Here's the drawing with two shaded views (mm, measured from the low corner). I have some questions. A direction names the side the tool comes from. Give positions to 0.01 mm unless a question says otherwise; leave off trailing zeros. Write each loop counter-clockwise with the first axis right and the second up, starting at its lowest first coordinate (ties: lowest second). Pieces come first, ordered by that corner, then holes. Notation, with made-up numbers: M 52,-18.75 L 71,-18.75 A16 cw 71,-13.75 Z; hole C -19,73.5 d10. An arc over 180 degrees is marked long. Answer as a JSON object with one key per item and string values. Group by question number.
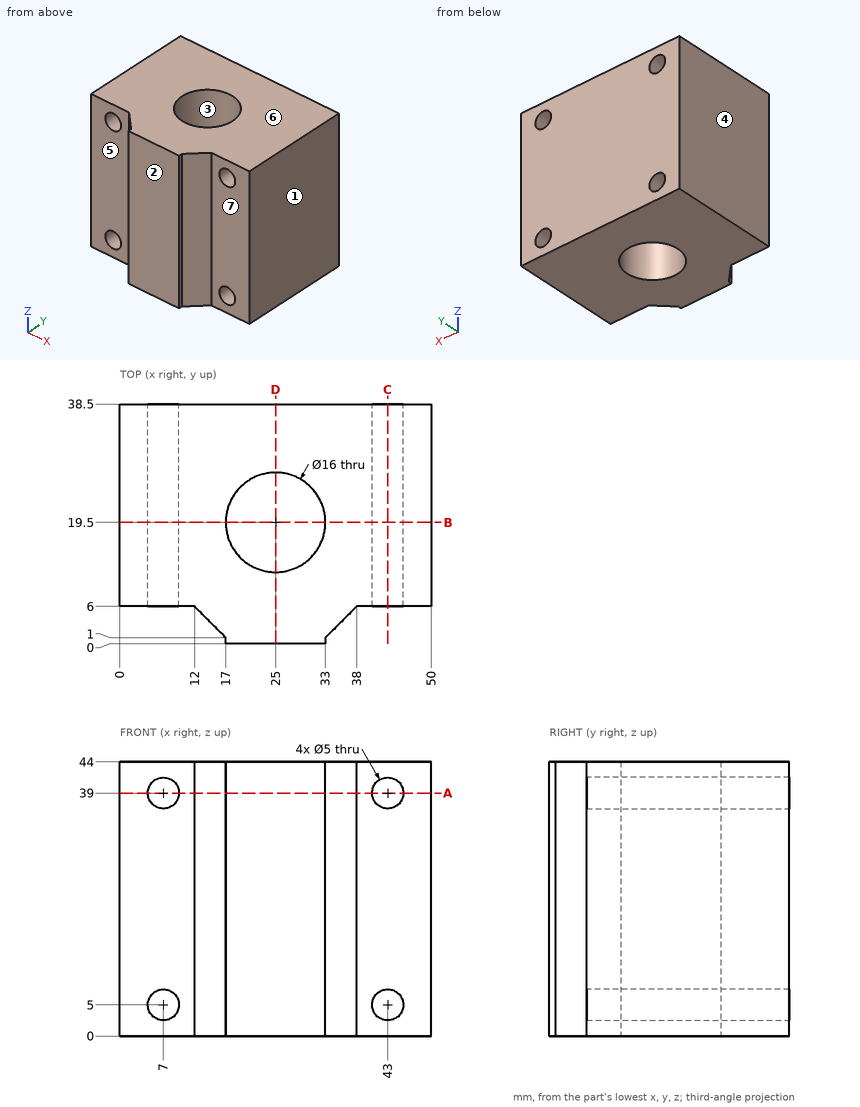
1) Please list where these lines run through material, in increasing order: line 1 along X through (y, z) = (31, 39); line 2 along X through (y, z) = (25, 39); line 3 along X through (y, z) = (18, 39.5). Write a range as from..to.
2) We'd pull the mould along X, two halves only. Please class the marked faces 1, 2, 3 and 4: released by +X, released by -X, zero draft, split by the parting line, or undercut.
3) For the marked faces 5, 6 and 7, which set-ups out of +Z, -Z, +X, -X, +Y, -Y let a thin tool reach every point of the face, with its end or its side?
4) I'm going to push flat-ended pins straight in: pin 1 (0.8 mm diameter, centred on y = 0.5, z = 24, fed in from -X); pin 2 (0.5 mm diameter, centred on y = 0.5, z = 30, fed in from +X); pin 3 (13 mm diameter, centred on x = 41.5, z = 11.5, fed in from -Y). Where does each tip first touch, or does it pass through?
5) If we section it at A-A, the plane z = 39: List the corners of the cut face in (x, y) for me, plus the area to 3 significant figures.
6) If we section it at D-D, the plane x = 25: List the corners of the cut face in (y, z) for me.
7) If we section it at B-B, the plane y = 19.5: List the corners of the cut face in (x, z) for me.
8) If we section it at C-C, the plane x = 43: List the corners of the cut face in (y, z) for me.
Taken from the geometry:
{
 "1": {"line 1": "0..4.5, 9.5..40.5, 45.5..50", "line 2": "0..4.5, 9.5..19.19, 30.81..40.5, 45.5..50", "line 3": "0..4.55, 9.45..17.14, 32.86..40.55, 45.45..50"},
 "2": {"face 1": "released by +X", "face 2": "zero draft", "face 3": "undercut", "face 4": "released by -X"},
 "3": {"face 5": "+Z, -Z, -X, -Y", "face 6": "+Z, +X, -X, +Y, -Y", "face 7": "+Z, -Z, +X, -Y"},
 "4": {"pin 1": "x = 17", "pin 2": "x = 33", "pin 3": "y = 3"},
 "5": {"outline": "M 0,6 L 4.5,6 L 4.5,38.5 L 0,38.5 Z; M 9.5,6 L 12,6 L 17,1 L 17,0 L 33,0 L 33,1 L 38,6 L 40.5,6 L 40.5,38.5 L 9.5,38.5 Z; M 45.5,6 L 50,6 L 50,38.5 L 45.5,38.5 Z; hole C 25,19.5 d16", "area": "1,220 mm²"},
 "6": {"outline": "M 0,0 L 11.5,0 L 11.5,44 L 0,44 Z; M 27.5,0 L 38.5,0 L 38.5,44 L 27.5,44 Z"},
 "7": {"outline": "M 0,0 L 17,0 L 17,44 L 0,44 Z; M 33,0 L 50,0 L 50,44 L 33,44 Z; hole C 7,5 d5; hole C 7,39 d5; hole C 43,5 d5; hole C 43,39 d5"},
 "8": {"outline": "M 6,0 L 38.5,0 L 38.5,2.5 L 6,2.5 Z; M 6,7.5 L 38.5,7.5 L 38.5,36.5 L 6,36.5 Z; M 6,41.5 L 38.5,41.5 L 38.5,44 L 6,44 Z"}
}
